from build123d import *

# Parameters (mm, degrees)
F0_R     = 11.1125
F0_R_2   = 7.9375
F1_DEPTH = 67.7418
F2_DEPTH = 28.575
F3_DEPTH = 28.575
F4_R     = 1.7272
F5_DEPTH = 12.1125001


with BuildPart() as f1:
    # F0 (on Top) → F1 (new body)
    with BuildSketch(Plane.XY):
        Circle(F0_R)
        Circle(F0_R_2, mode=Mode.SUBTRACT)
    extrude(amount=F1_DEPTH)

    # F2 (add): a face of the model
    f2_faces = [f1.faces().sort_by_distance(p)[0] for p in [
        (-10.7981910358, 0, 67.7418),
    ]]
    extrude(f2_faces, amount=F2_DEPTH)

    # F3 (add): a face of the model
    f3_faces = [f1.faces().sort_by_distance(p)[0] for p in [
        (-10.7981910358, 0, 0),
    ]]
    extrude(f3_faces, amount=F3_DEPTH)

    # F4 (on Front) → F5 (cut, up to face)
    with BuildSketch(Plane.XZ):
        with Locations((0, 33.8709)):
            Circle(F4_R)
        with Locations((0, 82.0293)):
            Circle(F4_R)
        with Locations((0, -14.2875)):
            Circle(F4_R)
    extrude(amount=-F5_DEPTH, mode=Mode.SUBTRACT)


solid = f1.part
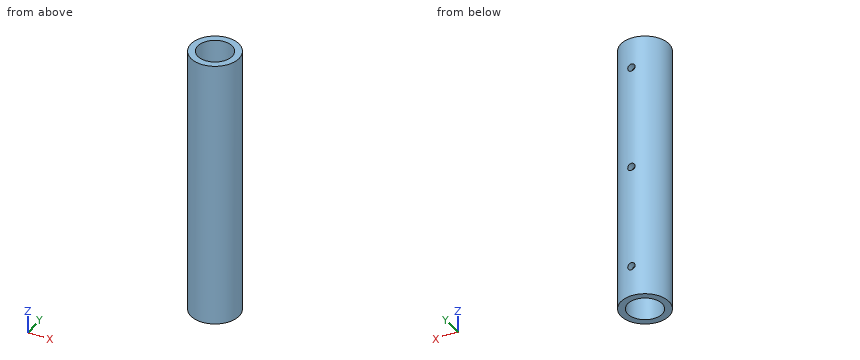
For this review, take the finished solid that the model builds, in its own axes (mm). Give positions to 0.01 mm unless a question says otherwise; leave off trailing zeros. Loops run counter-clockwise (first coordinate to the right, second up) from the corner with the lowest first, then second, coordinate; pieces in that order, holes last. Notation, with made-up numbers: (60.5, -36.5) - (65.5, -36.5) arc R11 ccw to (65.5, -24.5) - close; hole circle Ø5 at (-17.75, 13). An arc over 180 degrees is marked (long way). Write each question's results on one line, items separated by ' | '.
(1) Take a section at A-A (x = 0). Give the boundary of the cut face in (y, z) (1 decimal).
Conclusion:
outline: (-11.1, -28.6) - (-7.9, -28.6) - (-7.9, 96.3) - (-11.1, 96.3) - close; (7.9, -28.6) - (11.1, -28.6) - (11.1, -16) - (7.9, -16) - close; (7.9, -12.6) - (11.1, -12.6) - (11.1, 32.1) - (7.9, 32.1) - close; (7.9, 35.6) - (11.1, 35.6) - (11.1, 80.3) - (7.9, 80.3) - close; (7.9, 83.8) - (11.1, 83.8) - (11.1, 96.3) - (7.9, 96.3) - close
(2) Take a section at B-B (y = -6). Give the boundary of the cut face in (x, z) (3 decimals), then the cut area to 3 significant figures.
Conclusion:
outline: (-9.353, -28.575) - (-5.197, -28.575) - (-5.197, 96.317) - (-9.353, 96.317) - close; (5.197, -28.575) - (9.353, -28.575) - (9.353, 96.317) - (5.197, 96.317) - close | area: 1,040 mm^2
(3) Take a section at D-D (y = 0). Give the boundary of the cut face in (x, z) (1 decimal).
Conclusion:
outline: (-11.1, -28.6) - (-7.9, -28.6) - (-7.9, 96.3) - (-11.1, 96.3) - close; (7.9, -28.6) - (11.1, -28.6) - (11.1, 96.3) - (7.9, 96.3) - close
(4) For line 1 along Z through (x, y) = (0, 9.95) (1 decimal); line 2 along Y through (x, z) = (0, 74); line 3 along X through (y, z) = (0.5, 55.5), list the stretches that pass through material, from the lowest coordinate up.
Conclusion:
line 1: -28.6 to -16, -12.6 to 32.1, 35.6 to 80.3, 83.8 to 96.3 | line 2: -11.11 to -7.94, 7.94 to 11.11 | line 3: -11.1 to -7.92, 7.92 to 11.1
(5) Take a section at C-C (z = -2). Give the boundary of the cut face in (x, y) (1 decimal).
Conclusion:
outline: circle Ø22.2 at (0, 0); hole circle Ø15.9 at (0, 0)
(6) For pin 1 Ø6 at (x, z) = (-4, 83.5) entering from -Y; pin 2 Ø12.5 at (x, y) = (0, 0) entering from -Z; pin 3 Ø1.5 at (y, z) = (-5.5, 2) entering from -X; pin 4 Ø8 at (x, z) = (-6, 2) entering from +Y, all flat-tipped, find the tip position at first contact; note any pin that passes through.
Conclusion:
pin 1: y = -11.07 | pin 2: through | pin 3: x = -10.05 | pin 4: y = 10.93
